Autodesk Inventor part; units mm, degrees
ref_plane "YZ Plane" through (0, 0, 0) normal (1, 0, 0) x (0, 1, 0)
ref_plane "XZ Plane" through (0, 0, 0) normal (0, 1, 0) x (-1, 0, 0)
ref_plane "XY Plane" through (0, 0, 0) normal (0, 0, 1) x (1, 0, 0)
sketch "Sketch4" plane through (0, 0, 0) normal (0, 0, 1) x (1, 0, 0)
  line L0 (75, -100) -> (-75, -100)
  line L1 (-75, -100) -> (-75, 100)
  line L2 (-75, 100) -> (75, 100)
  line L3 (75, 100) -> (75, -100)
  line L4 (75, -100) -> (-75, 100) construction
  line L5 (-75, -100) -> (75, 100) construction
  line L6 (170, -37) -> (-170, -37)
  line L7 (-170, -37) -> (-170, 37)
  line L8 (-170, 37) -> (170, 37)
  line L9 (170, 37) -> (170, -37)
  line L10 (170, -37) -> (-170, 37) construction
  line L11 (-170, -37) -> (170, 37) construction
  point P0 (0, 0)
  point P1 (0, 0)
  point P2 (0, 0)
  point P3 (75, 37)
  point P4 (-75, 37)
  point P5 (-75, -37)
  point P6 (75, -37)
  dimension "d17" = 74
  dimension "d18" = 340
  dimension "d19" = 150
  dimension "d20" = 200
extrude "Extrusion4" add sketch "Sketch4" along normal mid plane 85
sketch "Sketch5" plane through (0, 0, 0) normal (0, 1, 0) x (-1, 0, 0)
  circle A0 centre (-125, 0) radius 39.5
  circle A1 centre (125, 0) radius 39.5
  line L0 (75, 42.5) -> (-75, 42.5) construction
  line L1 (0, 42.5) -> (0, -42.5) construction
  line L2 (-75, -42.5) -> (75, -42.5) construction
  line L3 (-170, -42.5) -> (-170, 42.5) construction
  line L4 (-170, 0) -> (170, 0) construction
  line L5 (170, -42.5) -> (170, 42.5) construction
  circle A2 centre (-125, 0) radius 31.5
  circle A3 centre (125, 0) radius 31.5
  line L6 (-155, 42.5) -> (-170, 27.5)
  line L7 (-170, -27.5) -> (-155, -42.5)
  line L8 (-170, -42.5) -> (-75, -42.5)
  line L9 (170, 42.5) -> (75, 42.5)
  line L10 (155, 42.5) -> (170, 27.5)
  line L11 (170, -27.5) -> (155, -42.5)
  line L12 (-75, 42.5) -> (-170, 42.5)
  line L13 (75, -42.5) -> (170, -42.5)
  line L14 (-170, 42.5) -> (-170, -42.5)
  line L15 (170, 42.5) -> (170, -42.5)
  circle A4 centre (125, 0) radius 25
  circle A5 centre (-125, 0) radius 25
  point P0 (0, 0)
  point P1 (-170, -27.5)
  dimension "d23" = 79
  dimension "d24" = 250
  dimension "d39" = 63
  dimension "d42" = 15
  dimension "d43" = 45
  dimension "d47" = 50
extrude "Extrusion5" add sketch "Sketch5" against normal blind 32 from surface at -37 contours A0 | A1 | A2 | A3 | A4 | A5
sketch "Sketch6" plane through (0, 0, 0) normal (0, 0, 1) x (1, 0, 0)
  line L0 (147, 10) -> (-147, 10)
  line L1 (-147, 10) -> (-147, -10)
  line L2 (-147, -10) -> (147, -10)
  line L3 (147, -10) -> (147, 10)
  line L4 (147, 10) -> (-147, -10) construction
  line L5 (-147, 10) -> (147, -10) construction
  line L6 (-60, 85) -> (60, 85)
  line L7 (60, 85) -> (60, -85)
  line L8 (60, -85) -> (-60, -85)
  line L9 (-60, -85) -> (-60, 85)
  line L10 (-60, 85) -> (60, -85) construction
  line L11 (60, 85) -> (-60, -85) construction
  line L12 (75, -100) -> (-75, -100)
  line L13 (-75, 37) -> (-75, 100)
  line L14 (-170, -37) -> (-170, 37)
  line L15 (-75, -37) -> (-170, -37)
  point P0 (0, 0)
  point P1 (-60, -10)
  point P2 (60, -10)
  point P3 (60, 10)
  point P4 (-60, 10)
  dimension "d27" = 15
  dimension "d28" = 15
  dimension "d29" = 23
  dimension "d30" = 27
  dimension "d46" = 20
extrude "Extrusion6" cut sketch "Sketch6" along normal mid plane 55
extrude "Extrusion8" cut sketch "Sketch5" against normal through all both and the other way through all contours L7 L8 L14 | L6 L14 L12 | L15 L10 L9 | L15 L13 L11
mirror "Mirror1" about plane through (0, 0, 0) normal (0, 1, 0) of "Extrusion5"
equation "\"d21\" = body_thickness"
equation "\"d27\" = wall_thickness"
equation "\"d28\" = wall_thickness"
equation "\"d31\" = body_thickness - 2 * wall_thickness"
equation "\"wall_thickness\" = 15"
equation "\"body_thickness\" = 85"
properties part number "body_inventor"
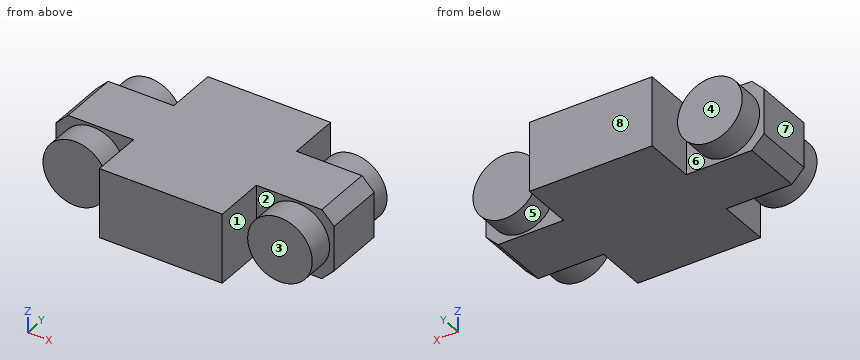
For this review, take the finished solid that the model builds, in its own axes (mm). Face numbers are marked on the shaded views. A direction names the side the tool comes from. Round coordinates to 2 decimals unless told otherwise and drop trailing zeros. Write each loop counter-clockwise with the first axis right and the second up, starting at its lowest first coordinate (ties: lowest second). Pieces come first, ordered by that corner, then holes. Notation, with made-up numbers: M -16,71.25 L 6,71.25 A20 ccw 6,94.25 Z; hole C 49,6 d6. An arc over 180 degrees is marked long. Write item = value, one per line. Start each with the question number.
(1) The part is to be moulded in two halves that separate along X. For the marked faces 6, 7 and 8, say which applies: +X half, -X half, draft (parallel to the pull), parting line (faces both ways), or undercut.
(2) We need section D-D (z = -31). Give the boundary of the cut face in (x, y).
(3) Clearance check with flat-ended pins moving along their axes: pin 1 Ø4 at (y, z) = (-62, -7) entering from +X; pin 2 Ø16.5 at (x, z) = (107.5, -11.5) entering from -Y; pin 3 Ø3 at (x, z) = (97.5, -25.5) entering from +Y. State where each tip first meets the part, or that it passes through.
(4) For line 1 along X through (y, z) = (68.5, 0.5); line 2 along X through (y, z) = (-80.5, -5.5); line 3 along Y through (x, z) = (112.5, -7), list the stretches that pass through material, from the lowest coordinate up.
(5) We need section C-C (y = 15.5). Give the boundary of the cut face in (x, z), then the cut area to 4 significant figures.
(6) We need section B-B (x = 19). Give the boundary of the cut face in (y, z).
(7) We need section A-A (y = 41). Give the boundary of the cut face in (x, z), then the cut area to 3 significant figures.
(8) For the marked faces 1, 2, 3, 4 and 5, list the 3-axis set-ups (+Z, -Z, +X, -X, +Y, -Y) from which the entire face can be reached by the end or side of a thin tool; tool diameter is ignored.
Results found:
q1.face_6 = undercut
q1.face_7 = -X half
q1.face_8 = draft
q2.outline = M -166.5,-37 L -149.48,-37 L -149.48,-69 L -100.52,-69 L -100.52,-37 L -75,-37 L -75,-100 L 75,-100 L 75,-37 L 100.52,-37 L 100.52,-69 L 149.48,-69 L 149.48,-37 L 166.5,-37 L 166.5,37 L 149.48,37 L 149.48,69 L 100.52,69 L 100.52,37 L 75,37 L 75,100 L -75,100 L -75,37 L -100.52,37 L -100.52,69 L -149.48,69 L -149.48,37 L -166.5,37 Z
q3.pin_1 = 164.18
q3.pin_2 = -69
q3.pin_3 = 69
q4.line_1 = -164.5 to -85.5, -75 to -60, 60 to 75, 85.5 to 164.5
q4.line_2 = -75 to -60, 60 to 75
q4.line_3 = -69 to -10, 10 to 69
q5.outline = M -170,-27.5 L -155,-42.5 L 155,-42.5 L 170,-27.5 L 170,27.5 L 155,42.5 L -155,42.5 L -170,27.5 Z; hole M -60,-27.5 L 60,-27.5 L 60,27.5 L -60,27.5 Z
q5.area = 21,850 mm²
q6.outline = M -100,-42.5 L 100,-42.5 L 100,42.5 L -100,42.5 Z; hole M -85,-27.5 L 85,-27.5 L 85,27.5 L -85,27.5 Z
q7.outline = C -125,0 d79; M -75,-42.5 L 75,-42.5 L 75,42.5 L -75,42.5 Z; C 125,0 d79; hole M -60,-27.5 L 60,-27.5 L 60,27.5 L -60,27.5 Z
q7.area = 16,000 mm²
q8.face_1 = +Z, -Z, -Y
q8.face_2 = -Y
q8.face_3 = +Z, -Z, +X, -Y
q8.face_4 = +Z, -Z, -X, +Y
q8.face_5 = +Y
